from build123d import *

# Parameters (mm, degrees)
SKETCH1_R                   = 10.25
SKETCH1_R_2                 = 3
BOSS_EXTRUDE1_DEPTH         = 2
IZIM1_R                     = 4
IZIM1_R_2                   = 3
Y_KSEKLIK_EKSTR_ZYON1_DEPTH = 4
KES_EKSTR_ZYON1_REACH       = 17.037
IZIM2_R                     = 0.625
DAIRESEL_O_ALTMA1_COUNT     = 4


with BuildPart() as part:
    # Sketch1 → Boss-Extrude1 (new body)
    with BuildSketch(Plane(origin=(0, 0, 0), x_dir=(1, 0, 0), z_dir=(0, 1, 0))):
        with Locations(Location((0, 0, 0), (0, 0, 270))):
            Circle(SKETCH1_R)
        with Locations(Location((0, 0, 0), (0, 0, 270))):
            Circle(SKETCH1_R_2, mode=Mode.SUBTRACT)
    extrude(amount=BOSS_EXTRUDE1_DEPTH)

    # izim1 → Y_kseklik-Ekstr_zyon1 (add)
    with BuildSketch(Plane(origin=(0, 2, 0), x_dir=(1, 0, 0), z_dir=(0, 1, 0))):
        with Locations(Location((0, 0, 0), (0, 0, 270))):
            Circle(IZIM1_R)
        with Locations(Location((0, 0, 0), (0, 0, 270))):
            Circle(IZIM1_R_2, mode=Mode.SUBTRACT)
    extrude(amount=Y_KSEKLIK_EKSTR_ZYON1_DEPTH)

    # izim2 → Kes-Ekstr_zyon1 (cut, up to next)
    with BuildSketch(Plane(origin=(0, 2, 0), x_dir=(1, 0, 0), z_dir=(0, 1, 0)), mode=Mode.PRIVATE) as kes_ekstr_zyon1_sk1:
        with Locations(Location((7.3, 0, 0), (0, 0, 270))):
            Circle(IZIM2_R)
    kes_ekstr_zyon1_tool1 = extrude(kes_ekstr_zyon1_sk1.sketch, amount=-KES_EKSTR_ZYON1_REACH, mode=Mode.PRIVATE) & part.part
    # izim2 → Kes-Ekstr_zyon1 (cut, up to next)
    with BuildSketch(Plane(origin=(0, 2, 0), x_dir=(1, 0, 0), z_dir=(0, 1, 0)), mode=Mode.PRIVATE) as kes_ekstr_zyon1_sk2:
        with Locations(Location((7.3, 3.75, 0), (0, 0, 270))):
            Circle(IZIM2_R)
    kes_ekstr_zyon1_tool2 = extrude(kes_ekstr_zyon1_sk2.sketch, amount=-KES_EKSTR_ZYON1_REACH, mode=Mode.PRIVATE) & part.part
    # izim2 → Kes-Ekstr_zyon1 (cut, up to next)
    with BuildSketch(Plane(origin=(0, 2, 0), x_dir=(1, 0, 0), z_dir=(0, 1, 0)), mode=Mode.PRIVATE) as kes_ekstr_zyon1_sk3:
        with Locations(Location((7.3, -3.75, 0), (0, 0, 270))):
            Circle(IZIM2_R)
    kes_ekstr_zyon1_tool3 = extrude(kes_ekstr_zyon1_sk3.sketch, amount=-KES_EKSTR_ZYON1_REACH, mode=Mode.PRIVATE) & part.part
    kes_ekstr_zyon1_1 = kes_ekstr_zyon1_tool1.solids().sort_by_distance((7.3, 2, 0))[0]
    add(kes_ekstr_zyon1_1, mode=Mode.SUBTRACT)
    kes_ekstr_zyon1_2 = kes_ekstr_zyon1_tool2.solids().sort_by_distance((7.3, 2, -3.75))[0]
    add(kes_ekstr_zyon1_2, mode=Mode.SUBTRACT)
    kes_ekstr_zyon1_3 = kes_ekstr_zyon1_tool3.solids().sort_by_distance((7.3, 2, 3.75))[0]
    add(kes_ekstr_zyon1_3, mode=Mode.SUBTRACT)
    kes_ekstr_zyon1 = kes_ekstr_zyon1_1 + kes_ekstr_zyon1_2 + kes_ekstr_zyon1_3  # Kes-Ekstr_zyon1 as one shape, for the pattern or mirror that repeats it

    # Dairesel _o_altma1: Kes-Ekstr_zyon1 ×4 about axis
    dairesel_o_altma1_axis = Axis((0, 0, 0), (0, 1, 0))
    for i in range(1, DAIRESEL_O_ALTMA1_COUNT):
        add(kes_ekstr_zyon1.rotate(dairesel_o_altma1_axis, i * 360 / DAIRESEL_O_ALTMA1_COUNT), mode=Mode.SUBTRACT)


solid = part.part
For this review, take the finished solid that the model builds, in its own axes (mm). Give positions to 0.01 mm unless a question says otherwise; leave off trailing zeros. Loops run counter-clockwise (first coordinate to the right, second up) from the corner with the lowest first, then second, coordinate; pieces in that order, holes last.
Item 1: For line 1 along X through (y, z) = (0.85, 3.75) (3 decimals); line 2 along X through (y, z) = (1.8, 4), list the stretches that pass through material, from the lowest coordinate up.
Item 2: Take a section at D-D, the plane x = -7.3. State the section outline as (y, z) points (3 decimals), and give its area (3 significant figures).
Item 3: Take a section at A-A, the plane z = 0. State the section outline as (x, y) points (3 decimals), and give its area (3 significant figures).
Item 4: Take a section at C-C, the plane x = -3.75. State the section outline as (y, z) points (3 decimals).
Item 5: Insertion check: pin 1 (0.8 mm diameter, centred on x = 3.75, z = -7.3, fed in from -Y); pin 2 (3 mm diameter, centred on x = 5.5, z = 7.5, fed in from +Y); pin 3 (3 mm diameter, centred on x = 4.5, y = 5, fed in from +Z). Each pin has a flat end and moves straight along its axis. Give the tip position at first contact, or say it passes through.
Item 6: Draft analysis for pull direction Z (two halves, no side actions). For faces 1 (the flat face through (0.1, 2, 4.4)), 2 (the cylindrical face through (6.92, 1.014, 3.254)), 3 (the cylindrical face through (-3.905, 3.972, -0.867)), state which applies: +Z half, -Z half, draft (parallel to the pull), parting line (faces both ways), or undercut.
Item 7: Take a section at B-B, the plane y = 0.95. Give the number of separate pieces and of enclosed holes in the cut face, and give its area (3 significant figures).
Calculated:
1. line 1: x = -9.539 to -7.925, -6.675 to 6.675, 7.925 to 9.539
1. line 2: x = -9.44 to -7.87, -6.73 to 6.73, 7.87 to 9.44
2. outline: (0, -7.195) - (2, -7.195) - (2, -4.375) - (0, -4.375) - close; (0, -3.125) - (2, -3.125) - (2, -0.625) - (0, -0.625) - close; (0, 0.625) - (2, 0.625) - (2, 3.125) - (0, 3.125) - close; (0, 4.375) - (2, 4.375) - (2, 7.195) - (0, 7.195) - close
2. area: 21.3 mm2
3. outline: (-10.25, 0) - (-7.925, 0) - (-7.925, 2) - (-10.25, 2) - close; (-6.675, 0) - (-3, 0) - (-3, 6) - (-4, 6) - (-4, 2) - (-6.675, 2) - close; (3, 0) - (6.675, 0) - (6.675, 2) - (4, 2) - (4, 6) - (3, 6) - close; (7.925, 0) - (10.25, 0) - (10.25, 2) - (7.925, 2) - close
3. area: 32.0 mm2
4. outline: (0, -9.539) - (2, -9.539) - (2, -7.925) - (0, -7.925) - close; (0, -6.675) - (2, -6.675) - (2, -1.392) - (6, -1.392) - (6, 1.392) - (2, 1.392) - (2, 6.675) - (0, 6.675) - close; (0, 7.925) - (2, 7.925) - (2, 9.539) - (0, 9.539) - close
5. pin 1: passes through
5. pin 2: stops at y = 2
5. pin 3: stops at z = 2.65
6. face 1: draft
6. face 2: undercut
6. face 3: parting line
7. separate pieces: 1
7. enclosed holes: 13
7. area: 287 mm2
